Autodesk Inventor part; units mm, degrees
ref_plane "YZ Plane" through (0, 0, 0) normal (1, 0, 0) x (0, 1, 0)
ref_plane "XZ Plane" through (0, 0, 0) normal (0, 1, 0) x (-1, 0, 0)
ref_plane "XY Plane" through (0, 0, 0) normal (0, 0, 1) x (1, 0, 0)
sketch "Sketch1" plane through (0, 0, 0) normal (0, 0, 1) x (1, 0, 0)
  arc A0 (45.111, 9) -> (-45.111, 9) centre (0, 0) ccw
  line L0 (35, 9) -> (35, 6)
  line L1 (35, 6) -> (25, 6)
  line L2 (25, 6) -> (25, 9)
  line L3 (-25, 9) -> (-25, 6)
  line L4 (-25, 6) -> (-35, 6)
  line L5 (-35, 6) -> (-35, 9)
  line L6 (-45.111, 9) -> (-35, 9)
  line L7 (-25, 9) -> (25, 9)
  line L8 (35, 9) -> (45.111, 9)
  line L9 (-22.2, 35.8) -> (-22.2, 30.2)
  line L10 (-22.2, 30.2) -> (-19.75, 30.2)
  line L11 (-19.75, 30.2) -> (-19.75, 28)
  line L12 (19.75, 28) -> (19.75, 30.2)
  line L13 (19.75, 30.2) -> (22.2, 30.2)
  line L14 (22.2, 30.2) -> (22.2, 35.8)
  line L15 (22.2, 35.8) -> (19.75, 35.8)
  line L16 (19.75, 35.8) -> (19.75, 38)
  line L17 (19.75, 38) -> (2, 38)
  line L18 (2, 38) -> (2, 39.6)
  line L19 (2, 39.6) -> (-2, 39.6)
  line L20 (-2, 39.6) -> (-2, 38)
  line L21 (-2, 38) -> (-19.75, 38)
  line L22 (-19.75, 38) -> (-19.75, 35.8)
  line L23 (-19.75, 35.8) -> (-22.2, 35.8)
  line L24 (-19.75, 28) -> (19.75, 28)
  line L25 (-15.5, 19) -> (-12.5, 19)
  line L26 (-12.5, 19) -> (-12.5, 14)
  line L27 (-12.5, 14) -> (-15.5, 14)
  line L28 (-15.5, 14) -> (-15.5, 19)
  line L29 (12.5, 19) -> (15.5, 19)
  line L30 (15.5, 19) -> (15.5, 14)
  line L31 (15.5, 14) -> (12.5, 14)
  line L32 (12.5, 14) -> (12.5, 19)
  circle A1 centre (0, 16.5) radius 5
  circle A2 centre (-28, 16.5) radius 5
  circle A3 centre (28, 16.5) radius 5
  dimension "d7" = 46
  dimension "d8" = 50
  dimension "d9" = 10
  dimension "d10" = 10
  dimension "d12" = 5.6
  dimension "d13" = 2.2
  dimension "d14" = 4
  dimension "d15" = 39.5
  dimension "d17" = 5.6
  dimension "d18" = 2.2
  dimension "d22" = 17.75
  dimension "d23" = 44.4
  dimension "d24" = 39.5
  dimension "d25" = 2.2
  dimension "d26" = 2.2
  dimension "d27" = 2.45
  dimension "d28" = 2.45
  dimension "d29" = 11.6
  dimension "d30" = 22.2
  dimension "d31" = 28
  dimension "d34" = 5
  dimension "d35" = 3
  dimension "d36" = 5
  dimension "d37" = 3
  dimension "d38" = 5
  dimension "d39" = 5
  dimension "d40" = 25
  dimension "d41" = 12.5
  dimension "d44" = 10
  dimension "d45" = 10
  dimension "d46" = 10
  dimension "d47" = 12.5
  dimension "d48" = 12.5
  dimension "d49" = 12.5
extrude "Extrusion3" add sketch "Sketch1" along normal blind 3
properties part number "OpenROV_Dev_EChassis_Plug_Mount"
Input: part model. Units: mm. Frame: model coordinates. A direction names the side the tool comes from. Coordinates: 2 decimals unless noted, no trailing zeros. Order: outer loops, then holes, each group sorted by start corner. A loop starts at its lowest first (then second) coordinate and runs counter-clockwise, first axis right, second up. Notation, with made-up numbers: (38.25, 59) - (83.25, 59) arc R22 ccw to (83.25, 71) - close; hole circle Ø6 at (80, -16). An arc over 180 degrees is marked (long way). Put each result on its own line as item: value.
1. Cut plane A-A on x = 0. Return the cut outline in (y, z), then the cut area to 3 significant figures.
Report:
outline: (9, 0) - (11.5, 0) - (11.5, 3) - (9, 3) - close; (21.5, 0) - (28, 0) - (28, 3) - (21.5, 3) - close; (39.6, 0) - (46, 0) - (46, 3) - (39.6, 3) - close
area: 46.2 mm2
2. Line query: line 1 along Y through (x, z) = (0, 2.25); line 2 along Y through (x, z) = (14.5, 2.45); line 3 along X through (y, z) = (18, 0.8). Output: solid intervals per line, ascending.
Report:
line 1: y = 9 to 11.5, 21.5 to 28, 39.6 to 46
line 2: y = 9 to 14, 19 to 28, 38 to 43.65
line 3: x = -42.33 to -32.77, -23.23 to -15.5, -12.5 to -4.77, 4.77 to 12.5, 15.5 to 23.23, 32.77 to 42.33
3. Cut plane D-D on z = 1.8. State how many separate pieces and enclosed holes the cut face has, then the cut area to 3 significant figures.
Report:
separate pieces: 1
enclosed holes: 6
area: 1,870 mm2
4. Reachability of faces 1 (the face through (40, 9, 1)), 2 (the face through (-35, 7, 1)), 3 (the face through (-25, 8, 1)), 4 (the face through (-0.88, 45.99, 1.48)), 5 (the face through (-15.5, 16, 1)) from +Z, -Z, +X, -X, +Y, -Y: full face, straight path, thin tool, end or side. Return the list, or none.
Report:
face 1: +Z, -Z, +X, -Y
face 2: +Z, -Z, -X, -Y
face 3: +Z, -Z, -Y
face 4: +Z, -Z, +Y
face 5: +Z, -Z
5. Contact query for flat-ended pins moving along their axis: pin 1 Ø1.1 at (y, z) = (28.5, 2) entering from +X; pin 2 Ø1.2 at (x, z) = (-21.5, 1) entering from +Y; pin 3 Ø1.5 at (y, z) = (12.5, 2.5) entering from +X; pin 4 Ø1 at (x, y) = (28.5, 19.5) entering from +Z. Output: stop coordinate, or through.
Report:
pin 1: stops at x = 36.53
pin 2: stops at y = 40.98
pin 3: stops at x = 44.47
pin 4: passes through
6. Cut plane C-C on y = 16.5. Return the cut outline in (x, z).
Report:
outline: (-42.94, 0) - (-33, 0) - (-33, 3) - (-42.94, 3) - close; (-23, 0) - (-15.5, 0) - (-15.5, 3) - (-23, 3) - close; (-12.5, 0) - (-5, 0) - (-5, 3) - (-12.5, 3) - close; (5, 0) - (12.5, 0) - (12.5, 3) - (5, 3) - close; (15.5, 0) - (23, 0) - (23, 3) - (15.5, 3) - close; (33, 0) - (42.94, 0) - (42.94, 3) - (33, 3) - close
7. Cut plane B-B on x = 31. Return the cut outline in (y, z).
Report:
outline: (6, 0) - (12.5, 0) - (12.5, 3) - (6, 3) - close; (20.5, 0) - (33.99, 0) - (33.99, 3) - (20.5, 3) - close
8. Draft query along Y for faces 6 (the face through (-12.5, 17, 1)), 7 (the face through (0, 28, 1)), 8 (the face through (-1, 26, 3)), 9 (the face through (-30, 6, 1)). Return one class per face: pulls with the +Y half, pulls with the -Y half, needs draft (parallel to the pull), parting line crosses it, or undercut.
Report:
face 6: undercut
face 7: undercut
face 8: needs draft
face 9: pulls with the -Y half
